Could you check a few things on this drawing? It's one solid part, dimensions in mm from its lowest x, y, z. A direction names the side the tool comes from. Give positions to 0.01 mm unless a question says otherwise; leave off trailing zeros. Loops run counter-clockwise (first coordinate to the right, second up) from the corner with the lowest first, then second, coordinate; pieces in that order, holes last. Notation, with made-up numbers: (87, -13) - (99, -13) arc R25 ccw to (99, 17) - close; hole circle Ø11 at (68, 9.5). An arc over 180 degrees is marked (long way). Use a Markdown table: item, result.
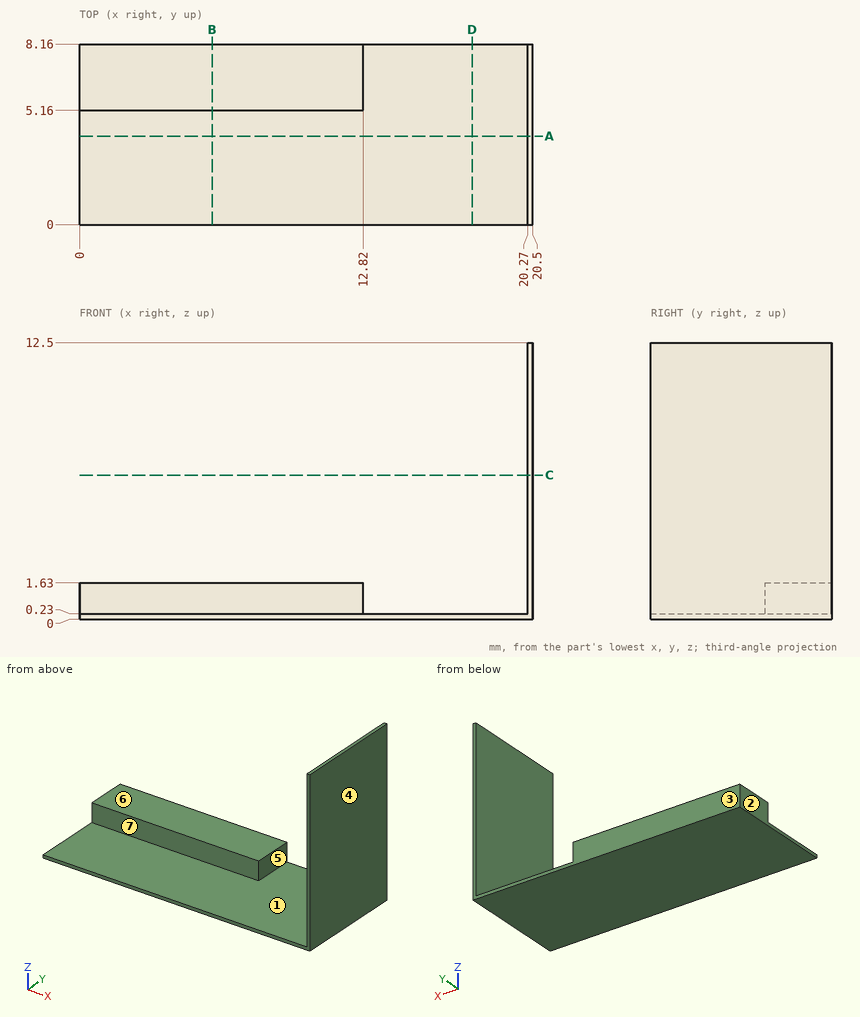
(1) Suppose I cut it at A-A on y = 4. Write out the boundary of the cut face in (x, z).
A:
| item | result |
|---|---|
| outline | (0, 0) - (20.5, 0) - (20.5, 12.5) - (20.27, 12.5) - (20.27, 0.23) - (0, 0.23) - close |
(2) If I drill on line 1 (X direction, y = 2.5, z = 4.5); line 2 (Z direction, x = 1.5, y = 6); line 3 (Z direction, x = 14, y = 3), over which ranges is the centre line in solid material (lowest first)?
A:
| item | result |
|---|---|
| line 1 | 20.27 to 20.5 |
| line 2 | 0 to 1.63 |
| line 3 | 0 to 0.23 |
(3) Suppose I cut it at C-C on z = 6.5. Write out the boundary of the cut face in (x, y).
A:
| item | result |
|---|---|
| outline | (20.27, 0) - (20.5, 0) - (20.5, 8.16) - (20.27, 8.16) - close |
(4) Suppose I cut it at D-D on x = 17.75. Write out the boundary of the cut face in (y, z), plus the area to 3 significant figures.
A:
| item | result |
|---|---|
| outline | (0, 0) - (8.16, 0) - (8.16, 0.23) - (0, 0.23) - close |
| area | 1.88 mm2 |
(5) We'd pull the mould along X, two halves only. Please class the marked faces 1, 2, 3 and 4: pulls with the +X half, pulls with the -X half, needs draft (parallel to the pull), parting line crosses it, or undercut.
A:
| item | result |
|---|---|
| face 1 | undercut |
| face 2 | pulls with the -X half |
| face 3 | needs draft |
| face 4 | pulls with the +X half |
(6) Will these pins go through, and if not, where does the flat tip stop? pin 1 (2.5 mm diameter, centred on y = 5.5, z = 7, fed in from -X); pin 2 (2.5 mm diameter, centred on x = 8.5, y = 6.5, fed in from +Z).
A:
| item | result |
|---|---|
| pin 1 | x = 20.27 |
| pin 2 | z = 1.63 |
(7) On a 3-axis mill with a long thin cutter (end or side, diameter ignored), from which of +Z, -Z, +X, -X, +Y, -Y can I reach the whole of each face in a straight line? I mean the marked faces 5, 6 and 7. Say none if no direction works.
A:
| item | result |
|---|---|
| face 5 | +Z, +Y, -Y |
| face 6 | +Z, -X, +Y, -Y |
| face 7 | +Z, -X, -Y |
(8) Suppose I cut it at B-B on x = 6. Write out the boundary of the cut face in (y, z).
A:
| item | result |
|---|---|
| outline | (0, 0) - (8.16, 0) - (8.16, 1.63) - (5.16, 1.63) - (5.16, 0.23) - (0, 0.23) - close |
